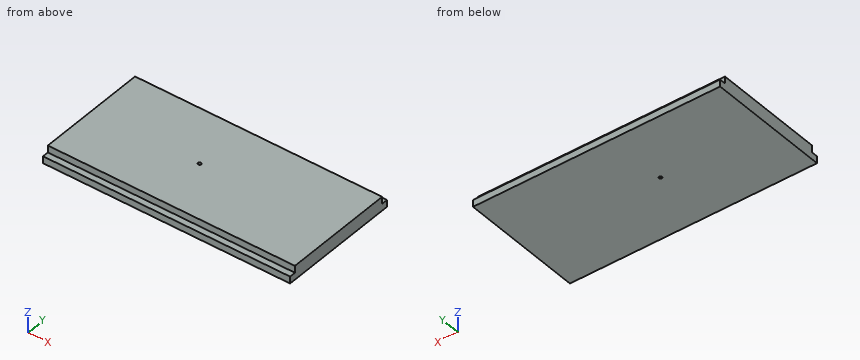
```python
from build123d import *

# Parameters (mm, degrees)
SKETCH1_W           = 40
SKETCH1_H           = 80
BOSS_EXTRUDE1_DEPTH = 4.5
SKETCH2_R           = 0.5
CUT_EXTRUDE1_DEPTH  = 90.555848497
SKETCH3_W           = 2
SKETCH3_H           = 2.25
CUT_EXTRUDE2_DEPTH  = 90.555848497


with BuildPart() as part:
    # Sketch1 → Boss-Extrude1 (new body)
    with BuildSketch(Plane(origin=(0, 0, 0), x_dir=(0, 1, 0), z_dir=(0, 0, 1))):
        with Locations((20, 40)):
            Rectangle(SKETCH1_W, SKETCH1_H)
    extrude(amount=BOSS_EXTRUDE1_DEPTH)

    # Sketch2 → Cut-Extrude1 (cut, through all)
    with BuildSketch(Plane.XY.offset(4.5)):
        with Locations((-45, 20)):
            Circle(SKETCH2_R)
    extrude(amount=-CUT_EXTRUDE1_DEPTH, mode=Mode.SUBTRACT)

    # Sketch3 → Cut-Extrude2 (cut, through all)
    with BuildSketch(Plane(origin=(-80, 0, 0), x_dir=(0, -1, 0), z_dir=(-1, 0, 0))):
        with Locations((-39, 3.375)):
            Rectangle(SKETCH3_W, SKETCH3_H)
        with Locations((-1, 3.375)):
            Rectangle(SKETCH3_W, SKETCH3_H)
    extrude(amount=-CUT_EXTRUDE2_DEPTH, mode=Mode.SUBTRACT)


solid = part.part
```
Source: CAD feature listing. Evaluate the final solid. Frame: model axes, mm. Coordinates: 2 decimals unless noted, no trailing zeros. Loops run counter-clockwise (first coordinate to the right, second up) from the corner with the lowest first, then second, coordinate; pieces in that order, holes last. Notation, with made-up numbers: M -3,68 L 46,68 A14 cw 46,78 Z; hole C 37,-7.5 d7. An arc over 180 degrees is marked long. Put each result on its own line as item: value. Start each with the question number.
1) Ray query, L1, parallel to Y at x = -45, z = 3.4; L2, parallel to Y at x = -45, z = 1.85; L3, parallel to Y at x = -62.5, z = 4.25. Return the intervals inside material, ascending. Write a range as from..to.
2) Cut plane A-A on x = -20. Return the cut outline in (y, z), then the cut area to 3 significant figures.
3) Contact query for flat-ended pins moving along their axis: pin 1 Ø0.6 at (x, y) = (-21.5, 38.5) entering from +Z; pin 2 Ø2.5 at (x, z) = (-24.5, 4) entering from +Y. Output: stop coordinate, or through.
The answers:
1. L1: y = 2..19.5, 20.5..38
1. L2: y = 0..19.5, 20.5..40
1. L3: y = 2..38
2. outline: M 0,0 L 40,0 L 40,2.25 L 38,2.25 L 38,4.5 L 2,4.5 L 2,2.25 L 0,2.25 Z
2. area: 171 mm²
3. pin 1: stops at z = 2.25
3. pin 2: stops at y = 38
